Source: CAD feature listing. Evaluate the final solid. Frame: model axes, mm. Face numbers are marked on the shaded views. A direction names the side the tool comes from. Give positions to 0.01 mm unless a question says otherwise; leave off trailing zeros. Order: outer loops, then holes, each group sorted by start corner. A loop starts at its lowest first (then second) coordinate and runs counter-clockwise, first axis right, second up. Notation, with made-up numbers: (17.5, -1.5) - (73.5, -1.5) arc R13 cw to (73.5, 14.5) - close; hole circle Ø1 at (36.5, 88). An arc over 180 degrees is marked (long way). One line per item, written item: value. Start each with the question number.
from build123d import *

# Parameters (mm, degrees)
BOSS_EXTRUDE1_DEPTH = 1.9558
SKETCH2_W           = 11.1506
SKETCH2_H           = 23.3426
BOSS_EXTRUDE2_DEPTH = 2.5019
SKETCH3_W           = 15.1892
SKETCH3_H           = 33.5026
BOSS_EXTRUDE3_DEPTH = 20.32
SKETCH4_R           = 10.9855
CUT_EXTRUDE1_DEPTH  = 40.489177087
SKETCH5_W           = 11.3792
SKETCH5_H           = 2.54
CUT_EXTRUDE2_DEPTH  = 44.289434312
FILLET1_R           = 1.27
SKETCH6_W           = 7.5692
SKETCH6_H           = 13.97
CUT_EXTRUDE3_DEPTH  = 1.27
SKETCH7_W           = 7.5692
SKETCH7_H           = 13.97
CUT_EXTRUDE4_DEPTH  = 1.27


with BuildPart() as part:
    # Sketch1 → Boss-Extrude1 (new body)
    with BuildSketch(Plane(origin=(0, 0, 0), x_dir=(1, 0, 0), z_dir=(0, 1, 0))):
        with BuildLine():
            Line((2.1971, 0), (12.9921, 0))
            ThreePointArc((12.9921, 0), (14.545684309, -0.643515691), (15.1892, -2.1971))
            Line((15.1892, -2.1971), (15.1892, -21.1455))
            ThreePointArc((15.1892, -21.1455), (14.545684309, -22.699084309), (12.9921, -23.3426))
            Line((12.9921, -23.3426), (2.1971, -23.3426))
            ThreePointArc((2.1971, -23.3426), (0.643515691, -22.699084309), (0, -21.1455))
            Line((0, -21.1455), (0, -2.1971))
            ThreePointArc((0, -2.1971), (0.643515691, -0.643515691), (2.1971, 0))
        make_face()
    extrude(amount=BOSS_EXTRUDE1_DEPTH)

    # Sketch2 → Boss-Extrude2 (add)
    with BuildSketch(Plane.XZ):
        with Locations((7.5946, 11.6713)):
            Rectangle(SKETCH2_W, SKETCH2_H)
    extrude(amount=BOSS_EXTRUDE2_DEPTH)

    # Sketch3 → Boss-Extrude3 (add)
    with BuildSketch(Plane.XZ.offset(2.5019)):
        with Locations((7.5946, 11.6713)):
            Rectangle(SKETCH3_W, SKETCH3_H)
    extrude(amount=BOSS_EXTRUDE3_DEPTH)

    # Sketch4 → Cut-Extrude1 (cut, through all)
    with BuildSketch(Plane(origin=(15.1892, 0, 0), x_dir=(0, 0, -1), z_dir=(1, 0, 0))):
        with Locations((-11.6713, -22.8219)):
            Circle(SKETCH4_R)
    extrude(amount=-CUT_EXTRUDE1_DEPTH, mode=Mode.SUBTRACT)

    # Sketch5 → Cut-Extrude2 (cut, through all)
    with BuildSketch(Plane.XY.offset(28.4226)):
        with Locations((7.5946, -7.5819)):
            Rectangle(SKETCH5_W, SKETCH5_H)
    extrude(amount=-CUT_EXTRUDE2_DEPTH, mode=Mode.SUBTRACT)

    # Fillet1
    fillet1_edges = [part.edges().sort_by_distance(p)[0] for p in [
        (13.2842, -8.8519, 11.6713),
        (13.2842, -6.3119, 11.6713),
        (1.905, -6.3119, 11.6713),
        (1.905, -8.8519, 11.6713),
    ]]
    fillet(fillet1_edges, radius=FILLET1_R - 0.0001)  # a hair under: the kernel refuses the full size

    # Sketch6 → Cut-Extrude3 (cut)
    with BuildSketch(Plane(origin=(0, 0, -5.08), x_dir=(-1, 0, 0), z_dir=(0, 0, -1))):
        with Locations((-7.5946, -15.8369)):
            Rectangle(SKETCH6_W, SKETCH6_H)
    extrude(amount=-CUT_EXTRUDE3_DEPTH, mode=Mode.SUBTRACT)

    # Sketch7 → Cut-Extrude4 (cut)
    with BuildSketch(Plane.XY.offset(28.4226)):
        with Locations((7.5946, -15.8369)):
            Rectangle(SKETCH7_W, SKETCH7_H)
    extrude(amount=-CUT_EXTRUDE4_DEPTH, mode=Mode.SUBTRACT)


solid = part.part
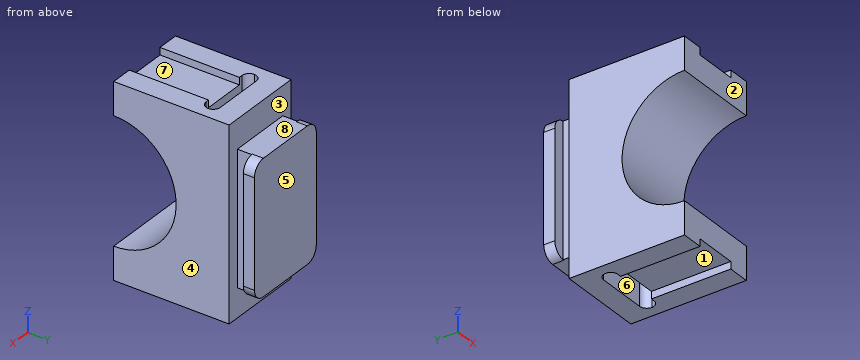
1. Set-up query: the marked faces 4, 5, 6, 7 and 8. Return all of +Z, -Z, +X, -X, +Y, -Y with unobstructed straight access to the full face (end or side cutting, diameter ignored); none if empty.
2. Section B-B on y = -14.25. Return the cut outline in (x, z).
3. Draft query along Y for the marked faces 1, 2 and 3. Return one class per face: pulls with the +Y half, pulls with the -Y half, needs draft (parallel to the pull), parting line crosses it, or undercut.
4. Contact query for flat-ended pins moving along their axis: pin 1 Ø0.6 at (y, z) = (-15.5, 28) entering from -X; pin 2 Ø6 at (x, y) = (7, -15.5) entering from +Z; pin 3 Ø1 at (x, z) = (1.5, 6) entering from -Y; pin 4 Ø0.8 at (y, z) = (-0.5, 7) entering from -X. Output: stop coordinate, or through.
5. Ray query, L1, parallel to Y at x = 5.5, z = 23.5; L2, parallel to Y at x = 14, z = 23.5; L3, parallel to Z at x = 7.5, y = -17.25. Return the intervals inside material, ascending.
Data:
1. face 4: +Z, -Z, +X, +Y, -Y
1. face 5: +Z, -Z, +X, -X, +Y
1. face 6: +Z, -Z
1. face 7: +Z, -Y
1. face 8: +Z, +X, -X, +Y
2. outline: (0, -5.08) - (3.81, -5.08) - (3.81, -3.81) - (11.38, -3.81) - (11.38, -5.08) - (15.19, -5.08) - (15.19, 4.8) - (0, 4.8) - close; (0, 18.54) - (15.19, 18.54) - (15.19, 28.42) - (11.38, 28.42) - (11.38, 27.15) - (3.81, 27.15) - (3.81, 28.42) - (0, 28.42) - close
3. face 1: needs draft
3. face 2: pulls with the -Y half
3. face 3: undercut
4. pin 1: stops at x = 0
4. pin 2: stops at z = 27.15
4. pin 3: stops at y = -13.73
4. pin 4: stops at x = 2.02
5. L1: y = -22.82 to -8.85, -6.31 to -2.5
5. L2: y = -22.82 to -2.5
5. L3: z = -3.81 to 2.2, 21.14 to 27.15
